from build123d import *

# Parameters (mm, degrees)
SKETCH1_R           = 14
BOSS_EXTRUDE1_DEPTH = 5
SKETCH2_R           = 10
BOSS_EXTRUDE2_DEPTH = 7
SKETCH3_R           = 1.5
CUT_EXTRUDE1_DEPTH  = 24.151673806
CUT_EXTRUDE2_REACH  = 25.152
SKETCH4_R           = 1.5


with BuildPart() as part:
    # Sketch1 → Boss-Extrude1 (new body)
    with BuildSketch(Plane.XY):
        Circle(SKETCH1_R)
    extrude(amount=BOSS_EXTRUDE1_DEPTH)

    # Sketch2 → Boss-Extrude2 (add)
    with BuildSketch(Plane.XY.offset(5)):
        Circle(SKETCH2_R)
    extrude(amount=BOSS_EXTRUDE2_DEPTH)

    # Sketch3 → Cut-Extrude1 (cut, through all)
    with BuildSketch(Plane.XY.offset(12)):
        Circle(SKETCH3_R)
    extrude(amount=-CUT_EXTRUDE1_DEPTH, mode=Mode.SUBTRACT)

    # Sketch4 → Cut-Extrude2 (cut, up to next)
    with BuildSketch(Plane.XY.offset(12), mode=Mode.PRIVATE) as cut_extrude2_sk1:
        with Locations((-5.699704026, 0)):
            Circle(SKETCH4_R)
    cut_extrude2_tool1 = extrude(cut_extrude2_sk1.sketch, amount=-CUT_EXTRUDE2_REACH, mode=Mode.PRIVATE) & part.part
    # Sketch4 → Cut-Extrude2 (cut, up to next)
    with BuildSketch(Plane.XY.offset(12), mode=Mode.PRIVATE) as cut_extrude2_sk2:
        with Locations((6.316954824, 0)):
            Circle(SKETCH4_R)
    cut_extrude2_tool2 = extrude(cut_extrude2_sk2.sketch, amount=-CUT_EXTRUDE2_REACH, mode=Mode.PRIVATE) & part.part
    add(cut_extrude2_tool1.solids().sort_by_distance((-5.699704, 0, 12))[0], mode=Mode.SUBTRACT)
    add(cut_extrude2_tool2.solids().sort_by_distance((6.316955, 0, 12))[0], mode=Mode.SUBTRACT)


solid = part.part
Input: part model. Units: mm. Frame: model coordinates. Coordinates: 2 decimals unless noted, no trailing zeros. Order: outer loops, then holes, each group sorted by start corner. A loop starts at its lowest first (then second) coordinate and runs counter-clockwise, first axis right, second up. Notation, with made-up numbers: M 43,52 L 55,52 A19 cw 55,68 Z; hole C 68.25,56 d5. An arc over 180 degrees is marked long. Answer as CSV lines item,"result".
1. Material intervals for line 1 (Y direction, x = 0, z = 8); line 2 (X direction, y = 0.75, z = 5.5); line 3 (Y direction, x = 0, z = 4), sorted ascending. Write a range as from..to.
Reported:
line 1,"-10..-1.5, 1.5..10"
line 2,"-9.97..-7, -4.4..-1.3, 1.3..5.02, 7.62..9.97"
line 3,"-14..-1.5, 1.5..14"
2. Section D-D (y = 7). Return the cut outline in (x, z), then the cut area to 3 significant figures.
Reported:
outline,"M -12.12,0 L 12.12,0 L 12.12,5 L 7.14,5 L 7.14,12 L -7.14,12 L -7.14,5 L -12.12,5 Z"
area,"221 mm2"
3. Section A-A (y = 0). Return the cut outline in (x, z).
Reported:
outline,"M -14,0 L -7.2,0 L -7.2,12 L -10,12 L -10,5 L -14,5 Z; M -4.2,0 L -1.5,0 L -1.5,12 L -4.2,12 Z; M 1.5,0 L 4.82,0 L 4.82,12 L 1.5,12 Z; M 7.82,0 L 14,0 L 14,5 L 10,5 L 10,12 L 7.82,12 Z"
4. Section C-C (z = 6.5). Return the cut outline in (x, y), then the cut area to 3 significant figures.
Reported:
outline,"C 0,0 d20; hole C -5.7,0 d3; hole C 0,0 d3; hole C 6.32,0 d3"
area,"293 mm2"
5. First-contact query: P1, Ø6, axis at x = 3, z = 9, coming from the +Y side; P2, Ø5, axis at y = -4, z = 6, coming from the +X side. Flat tips, straight axial feed; report the tip coordinate or a pass-through.
Reported:
P1,"y = 10"
P2,"x = 13.9"
6. Pull-direction query (X, two-part tool) for faces 1 (the cylindrical face through (-4.27, 0.45, 6.08)), 2 (the flat face through (-3, 10, 5)), 3 (the cylindrical face through (-2.17, -9.76, 8.45)); classes: released by +X, released by -X, zero draft, split by the parting line, or undercut.
Reported:
face 1,"undercut"
face 2,"zero draft"
face 3,"split by the parting line"
7. Section B-B (x = 0). Return the cut outline in (y, z).
Reported:
outline,"M -14,0 L -1.5,0 L -1.5,12 L -10,12 L -10,5 L -14,5 Z; M 1.5,0 L 14,0 L 14,5 L 10,5 L 10,12 L 1.5,12 Z"
